Can you work these out from the model? Positions are in its coordinate system, mm. A direction names the side the tool comes from. Round coordinates to 2 decimals unless told otherwise and drop trailing zeros. Loops run counter-clockwise (first coordinate to the right, second up) from the corner with the lowest first, then second, coordinate; pieces in that order, holes last. Notation, with made-up numbers: (69.25, -5) -> (101.25, -5) arc R31 cw to (101.25, 29) -> close; hole circle Ø2 at (32.5, 74.5). An arc over 180 degrees is marked (long way). Write each question's results on one line, items separated by ' | '.
from build123d import *

# Parameters (mm, degrees)
F1_DEPTH = 25
F2_R     = 1.5
F3_R     = 1.5
F4_R     = 1.5
F5_DEPTH = 10


with BuildPart() as f1:
    # F0 (on Front) → F1 (new body, symmetric)
    with BuildSketch(Plane.XZ):
        with BuildLine():
            Line((-12.5, 2), (-12.5, 0))
            Line((-12.5, 0), (12.5, 0))
            Line((12.5, 0), (12.5, 2))
            Line((12.5, 2), (10.5, 2))
            ThreePointArc((10.5, 2), (5.9038059223, 3.9038059223), (4, 8.5))
            Line((4, 8.5), (4, 10.7250827824))
            ThreePointArc((4, 10.7250827824), (0, 20), (-4, 10.7250827824))
            Line((-4, 10.7250827824), (-4, 8.5))
            ThreePointArc((-4, 8.5), (-5.9038059223, 3.9038059223), (-10.5, 2))
            Line((-10.5, 2), (-12.5, 2))
        make_face()
    extrude(amount=F1_DEPTH, both=True)

    # F2
    f2_edges = [f1.edges().sort_by_distance(p)[0] for p in [
        (12.5, 0, 2),
        (-12.5, 0, 2),
    ]]
    fillet(f2_edges, radius=F2_R)

    # F3
    f3_edges = [f1.edges().sort_by_distance(p)[0] for p in [
        (0, -25, 20),
        (4, -25, 9.612541),
        (-4, -25, 9.612541),
        (0, 25, 20),
        (4, 25, 9.612541),
        (-5.903806, 25, 3.903806),
    ]]
    fillet(f3_edges, radius=F3_R)

    # F4 (on face) → F5 (cut)
    with BuildSketch(Plane(origin=(0, 0, 0), x_dir=(1, 0, 0), z_dir=(0, 0, -1))):
        Circle(F4_R)
        with Locations((0, 12)):
            Circle(F4_R)
        with Locations((0, -12)):
            Circle(F4_R)
    extrude(amount=-F5_DEPTH, mode=Mode.SUBTRACT)


solid = f1.part
1. On a 3-axis mill with a long thin cutter (end or side, diameter ignored), from which of +Z, -Z, +X, -X, +Y, -Y can I reach the whole of each face in a straight line? I mean faces 1 (the face through (-10.75, 24.57, 1.55)), 2 (the face through (-0.325, 13.464, 4.93)), 3 (the face through (-3.55, -24.57, 9.6)). Say none if no direction works.
Final values:
face 1: +Z, -X, +Y | face 2: -Z | face 3: -X, -Y
2. If we section it at D-D (y = 0.5): List the corners of the cut face in (x, z) for me, then the cut area to 3 significant figures.
Final values:
outline: (-12.5, 0) -> (-1.41, 0) -> (-1.41, 10) -> (1.41, 10) -> (1.41, 0) -> (12.5, 0) -> (12.5, 0.5) arc R1.5 ccw to (11, 2) -> (10.5, 2) arc R6.5 cw to (4, 8.5) -> (4, 10.73) arc R5.5 ccw (long way) to (-4, 10.73) -> (-4, 8.5) arc R6.5 cw to (-10.5, 2) -> (-11, 2) arc R1.5 ccw to (-12.5, 0.5) -> close | area: 194 mm2
3. Please list where these lines run through material, in increasing order: line 1 (Y direction, x = 0, z = 5.25); line 2 (X direction, y = 3, z = 9.25); line 3 (X direction, y = -23, z = 14.5). Write a range as from..to.
Final values:
line 1: -25..-13.5, -10.5..-1.5, 1.5..10.5, 13.5..25 | line 2: -4..4 | line 3: -5.5..5.5
4. If we section it at B-B (x = 0): List the corners of the cut face in (y, z) for me.
Final values:
outline: (-25, 0) -> (-13.5, 0) -> (-13.5, 10) -> (-10.5, 10) -> (-10.5, 0) -> (-1.5, 0) -> (-1.5, 10) -> (1.5, 10) -> (1.5, 0) -> (10.5, 0) -> (10.5, 10) -> (13.5, 10) -> (13.5, 0) -> (25, 0) -> (25, 18.5) arc R1.5 ccw to (23.5, 20) -> (-23.5, 20) arc R1.5 ccw to (-25, 18.5) -> close
5. If we section it at A-A (y = 12): List the corners of the cut face in (x, z) for me, then the cut area to 3 significant figures.
Final values:
outline: (-12.5, 0) -> (-1.5, 0) -> (-1.5, 10) -> (1.5, 10) -> (1.5, 0) -> (12.5, 0) -> (12.5, 0.5) arc R1.5 ccw to (11, 2) -> (10.5, 2) arc R6.5 cw to (4, 8.5) -> (4, 10.73) arc R5.5 ccw (long way) to (-4, 10.73) -> (-4, 8.5) arc R6.5 cw to (-10.5, 2) -> (-11, 2) arc R1.5 ccw to (-12.5, 0.5) -> close | area: 192 mm2
6. If we section it at C-C (y = -18): List the corners of the cut face in (x, z) for me, then the cut area to 3 significant figures.
Final values:
outline: (-12.5, 0) -> (12.5, 0) -> (12.5, 0.5) arc R1.5 ccw to (11, 2) -> (10.5, 2) arc R6.5 cw to (4, 8.5) -> (4, 10.73) arc R5.5 ccw (long way) to (-4, 10.73) -> (-4, 8.5) arc R6.5 cw to (-10.5, 2) -> (-11, 2) arc R1.5 ccw to (-12.5, 0.5) -> close | area: 222 mm2
7. Will these pins go through, and if not, where does the flat tip stop? pin 1 (2 mm diameter, centred on y = -11, z = 13.5, fed in from -X); pin 2 (0.6 mm diameter, centred on x = 11, y = 10, fed in from +Z); pin 3 (1.1 mm diameter, centred on y = -3, z = 10, fed in from +X).
Final values:
pin 1: x = -5.5 | pin 2: z = 2 | pin 3: x = 4
8. We'd pull the mould along Z, two halves only. Please class faces 4 (the face through (5.955, -0.329, 3.854)), 5 (the face through (-1, 25, 8)), 6 (the face through (0, -12, 10)): pulls with the +Z half, pulls with the -Z half, needs draft (parallel to the pull), parting line crosses it, or undercut.
Final values:
face 4: undercut | face 5: needs draft | face 6: pulls with the -Z half
